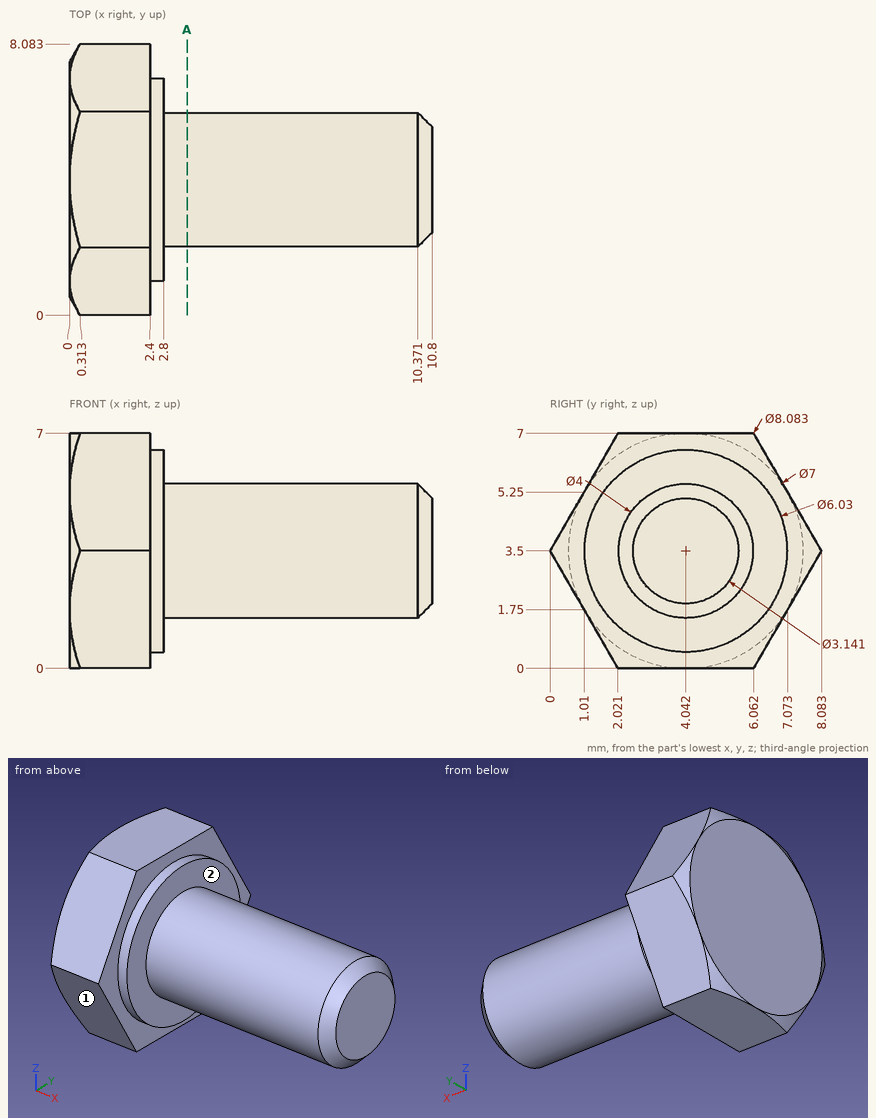
Answer from the drawing. Dimensions are ordinates in mm from the lowest x, y and z of the part. A direction names the side the tool comes from. Round coordinates to 2 decimals unless told otherwise and drop trailing zeros. Loops run counter-clockwise (first coordinate to the right, second up) from the corner with the lowest first, then second, coordinate; pieces in that order, holes last.
1) Consider line 1 (X direction, y = 7, z = 5); line 2 (Z direction, x = 2.25, y = 7) (1 decimal); line 3 (Y direction, x = 1, z = 6.5). Determine where each line is inside the solid, lowest interval first.
Outcome:
line 1: x = 0 to 2.4
line 2: z = 1.6 to 5.4
line 3: y = 1.73 to 6.35
2) For the marked faces 1 and 2, determine the directions among +Z, -Z, +X, -X, +Y, -Y from which every point of the face is accessible in a straight line to the end or side of a thin tool.
Outcome:
face 1: -Z, +X, -X, -Y
face 2: +X
3) Given P1, Ø2, axis at x = 7, y = 1, coming from the -Z side; P2, Ø4, axis at x = 6.5, z = 4.5, coming from the -Y side; P3, Ø3, axis at x = 9.5, z = 4.5, coming from the +Y side; P4, Ø1.5, axis at y = 2.5, z = 4, coming from the -X side, each flat-ended and moving along its own axis, determine where each tip first touches the part or whether it passes through.
Outcome:
P1: passes through
P2: stops at y = 2.04
P3: stops at y = 6.04
P4: stops at x = 0
4) A cutting plane is placed at A-A on x = 3.5. Determine the outline of the cut face in (y, z), plus the area to 3 significant figures.
Outcome:
outline: circle Ø4 at (4.04, 3.5)
area: 12.6 mm2
